```python
from build123d import *

# Parameters (mm, degrees)
EXTRUDE1_DEPTH                     = 2.5
SKETCH2_W                          = 1.54
SKETCH2_H                          = 0.508742985
CUT_EXTRUDE1_DEPTH                 = 12.5
SKETCH3_W                          = 0.65
SKETCH3_H                          = 0.65
EXTRUDE2_DEPTH                     = 3.54
CHAMFER1_SIZE                      = 0.35
CHAMFER1_SIZE2                     = 0.16320768
CHAMFER1_PART_2_SIZE               = 0.35
CHAMFER1_PART_2_SIZE2              = 0.16320768
CHAMFER1_PART_3_SIZE               = 0.35
CHAMFER1_PART_3_SIZE2              = 0.16320768
CHAMFER1_PART_4_SIZE               = 0.35
CHAMFER1_PART_4_SIZE2              = 0.16320768
SKETCH4_W                          = 0.65
SKETCH4_H                          = 0.65
EXTRUDE3_DEPTH                     = 6
CHAMFER2_SIZE                      = 0.35
CHAMFER2_SIZE2                     = 0.16320768
CHAMFER2_PART_2_SIZE               = 0.35
CHAMFER2_PART_2_SIZE2              = 0.16320768
CHAMFER2_PART_3_SIZE               = 0.35
CHAMFER2_PART_3_SIZE2              = 0.16320768
CHAMFER2_PART_4_SIZE               = 0.35
CHAMFER2_PART_4_SIZE2              = 0.16320768
LPATTERN3_COUNT                    = 2
LPATTERN3_PITCH                    = 2.54
LPATTERN3_COUNT_DIR2               = 2
LPATTERN3_PITCH_DIR2               = 2.54
LPATTERN4_COUNT                    = 2
LPATTERN4_PITCH                    = 2.54
LPATTERN4_COUNT_DIR2               = 2
LPATTERN4_PITCH_DIR2               = 2.54
CHAMFER1_OF_LPATTERN4_SIZE2        = 0.16320768
CHAMFER1_OF_LPATTERN4_SIZE         = 0.35
CHAMFER1_PART_2_OF_LPATTERN4_SIZE2 = 0.16320768
CHAMFER1_PART_2_OF_LPATTERN4_SIZE  = 0.35
CHAMFER1_PART_3_OF_LPATTERN4_SIZE2 = 0.16320768
CHAMFER1_PART_3_OF_LPATTERN4_SIZE  = 0.35
CHAMFER1_PART_4_OF_LPATTERN4_SIZE2 = 0.16320768
CHAMFER1_PART_4_OF_LPATTERN4_SIZE  = 0.35
CHAMFER2_OF_LPATTERN4_SIZE2        = 0.16320768
CHAMFER2_OF_LPATTERN4_SIZE         = 0.35
CHAMFER2_PART_2_OF_LPATTERN4_SIZE2 = 0.16320768
CHAMFER2_PART_2_OF_LPATTERN4_SIZE  = 0.35
CHAMFER2_PART_3_OF_LPATTERN4_SIZE2 = 0.16320768
CHAMFER2_PART_3_OF_LPATTERN4_SIZE  = 0.35
CHAMFER2_PART_4_OF_LPATTERN4_SIZE2 = 0.16320768
CHAMFER2_PART_4_OF_LPATTERN4_SIZE  = 0.35
ESBO_O1_R                          = 0.039608668
CORTE_EXTRUS_O1_DEPTH              = 0.1


with BuildPart() as part:
    # Sketch1 → Extrude1 (new body)
    with BuildSketch(Plane(origin=(0, 0, 0), x_dir=(1, 0, 0), z_dir=(0, 1, 0))):
        Polygon((-0.97, 1.27), (0.97, 1.27), (1.27, 0.97), (1.27, -0.97), (0.97, -1.27), (-0.97, -1.27), (-1.27, -0.97), (-1.27, 0.97), align=None)
    extrude1 = extrude(amount=EXTRUDE1_DEPTH)

    # Sketch2 → Cut-Extrude1 (cut)
    with BuildSketch(Plane.XY.offset(1.27)):
        with Locations((0, 2.314371493)):
            Rectangle(SKETCH2_W, SKETCH2_H)
    cut_extrude1 = extrude(amount=-CUT_EXTRUDE1_DEPTH, mode=Mode.SUBTRACT)

    # Sketch3 → Extrude2 (add)
    with BuildSketch(Plane(origin=(0, 2.06, 0), x_dir=(-1, 0, 0), z_dir=(0, 1, 0))):
        Rectangle(SKETCH3_W, SKETCH3_H)
    extrude2 = extrude(amount=EXTRUDE2_DEPTH)

    # Chamfer1
    chamfer1_edges = [part.edges().sort_by_distance(p)[0] for p in [
        (-0.325, 5.6, 0),
    ]]
    chamfer1_side = [part.faces().sort_by_distance(p)[0] for p in [
        (-0.325, 3.83, 0),
    ]]
    chamfer(chamfer1_edges, length=CHAMFER1_SIZE, length2=CHAMFER1_SIZE2, reference=chamfer1_side[0])

    # Chamfer1 part 2
    chamfer1_part_2_edges = [part.edges().sort_by_distance(p)[0] for p in [
        (0, 5.6, 0.325),
    ]]
    chamfer1_part_2_side = [part.faces().sort_by_distance(p)[0] for p in [
        (0, 3.83, 0.325),
    ]]
    chamfer(chamfer1_part_2_edges, length=CHAMFER1_PART_2_SIZE, length2=CHAMFER1_PART_2_SIZE2, reference=chamfer1_part_2_side[0])

    # Chamfer1 part 3
    chamfer1_part_3_edges = [part.edges().sort_by_distance(p)[0] for p in [
        (0.325, 5.6, 0),
    ]]
    chamfer1_part_3_side = [part.faces().sort_by_distance(p)[0] for p in [
        (0.325, 3.83, 0),
    ]]
    chamfer(chamfer1_part_3_edges, length=CHAMFER1_PART_3_SIZE, length2=CHAMFER1_PART_3_SIZE2, reference=chamfer1_part_3_side[0])

    # Chamfer1 part 4
    chamfer1_part_4_edges = [part.edges().sort_by_distance(p)[0] for p in [
        (0, 5.6, -0.325),
    ]]
    chamfer1_part_4_side = [part.faces().sort_by_distance(p)[0] for p in [
        (0, 3.83, -0.325),
    ]]
    chamfer(chamfer1_part_4_edges, length=CHAMFER1_PART_4_SIZE, length2=CHAMFER1_PART_4_SIZE2, reference=chamfer1_part_4_side[0])

    # Sketch4 → Extrude3 (add)
    with BuildSketch(Plane.XZ):
        Rectangle(SKETCH4_W, SKETCH4_H)
    extrude3 = extrude(amount=EXTRUDE3_DEPTH)

    # Chamfer2
    chamfer2_edges = [part.edges().sort_by_distance(p)[0] for p in [
        (-0.325, -6, 0),
    ]]
    chamfer2_side = [part.faces().sort_by_distance(p)[0] for p in [
        (-0.325, -3, 0),
    ]]
    chamfer(chamfer2_edges, length=CHAMFER2_SIZE, length2=CHAMFER2_SIZE2, reference=chamfer2_side[0])

    # Chamfer2 part 2
    chamfer2_part_2_edges = [part.edges().sort_by_distance(p)[0] for p in [
        (0, -6, -0.325),
    ]]
    chamfer2_part_2_side = [part.faces().sort_by_distance(p)[0] for p in [
        (0, -3, -0.325),
    ]]
    chamfer(chamfer2_part_2_edges, length=CHAMFER2_PART_2_SIZE, length2=CHAMFER2_PART_2_SIZE2, reference=chamfer2_part_2_side[0])

    # Chamfer2 part 3
    chamfer2_part_3_edges = [part.edges().sort_by_distance(p)[0] for p in [
        (0.325, -6, 0),
    ]]
    chamfer2_part_3_side = [part.faces().sort_by_distance(p)[0] for p in [
        (0.325, -3, 0),
    ]]
    chamfer(chamfer2_part_3_edges, length=CHAMFER2_PART_3_SIZE, length2=CHAMFER2_PART_3_SIZE2, reference=chamfer2_part_3_side[0])

    # Chamfer2 part 4
    chamfer2_part_4_edges = [part.edges().sort_by_distance(p)[0] for p in [
        (0, -6, 0.325),
    ]]
    chamfer2_part_4_side = [part.faces().sort_by_distance(p)[0] for p in [
        (0, -3, 0.325),
    ]]
    chamfer(chamfer2_part_4_edges, length=CHAMFER2_PART_4_SIZE, length2=CHAMFER2_PART_4_SIZE2, reference=chamfer2_part_4_side[0])

    # LPattern3: Extrude1, Cut-Extrude1 2 × 2
    with Locations(*[(-j * LPATTERN3_PITCH_DIR2, 0, -i * LPATTERN3_PITCH) for i in range(LPATTERN3_COUNT) for j in range(LPATTERN3_COUNT_DIR2) if (i, j) != (0, 0)]):
        add(extrude1)
        add(cut_extrude1, mode=Mode.SUBTRACT)

    # LPattern4: Extrude2, Extrude3 2 × 2
    with Locations(*[(-j * LPATTERN4_PITCH_DIR2, 0, -i * LPATTERN4_PITCH) for i in range(LPATTERN4_COUNT) for j in range(LPATTERN4_COUNT_DIR2) if (i, j) != (0, 0)]):
        add(extrude2)
        add(extrude3)

    # Chamfer1 of LPattern4
    chamfer1_of_lpattern4_edges = [part.edges().sort_by_distance(p)[0] for p in [
        (-2.865, 5.6, 0),
        (-0.325, 5.6, -2.54),
        (-2.865, 5.6, -2.54),
    ]]
    chamfer(chamfer1_of_lpattern4_edges, length=CHAMFER1_OF_LPATTERN4_SIZE, length2=CHAMFER1_OF_LPATTERN4_SIZE2)

    # Chamfer1 part 2 of LPattern4
    chamfer1_part_2_of_lpattern4_edges = [part.edges().sort_by_distance(p)[0] for p in [
        (-2.54, 5.6, 0.325),
        (0, 5.6, -2.215),
        (-2.54, 5.6, -2.215),
    ]]
    chamfer(chamfer1_part_2_of_lpattern4_edges, length=CHAMFER1_PART_2_OF_LPATTERN4_SIZE, length2=CHAMFER1_PART_2_OF_LPATTERN4_SIZE2)

    # Chamfer1 part 3 of LPattern4
    chamfer1_part_3_of_lpattern4_edges = [part.edges().sort_by_distance(p)[0] for p in [
        (-2.215, 5.6, 0),
        (0.325, 5.6, -2.54),
        (-2.215, 5.6, -2.54),
    ]]
    chamfer(chamfer1_part_3_of_lpattern4_edges, length=CHAMFER1_PART_3_OF_LPATTERN4_SIZE, length2=CHAMFER1_PART_3_OF_LPATTERN4_SIZE2)

    # Chamfer1 part 4 of LPattern4
    chamfer1_part_4_of_lpattern4_edges = [part.edges().sort_by_distance(p)[0] for p in [
        (-2.54, 5.6, -0.325),
        (0, 5.6, -2.865),
        (-2.54, 5.6, -2.865),
    ]]
    chamfer(chamfer1_part_4_of_lpattern4_edges, length=CHAMFER1_PART_4_OF_LPATTERN4_SIZE, length2=CHAMFER1_PART_4_OF_LPATTERN4_SIZE2)

    # Chamfer2 of LPattern4
    chamfer2_of_lpattern4_edges = [part.edges().sort_by_distance(p)[0] for p in [
        (-2.865, -6, 0),
        (-0.325, -6, -2.54),
        (-2.865, -6, -2.54),
    ]]
    chamfer(chamfer2_of_lpattern4_edges, length=CHAMFER2_OF_LPATTERN4_SIZE, length2=CHAMFER2_OF_LPATTERN4_SIZE2)

    # Chamfer2 part 2 of LPattern4
    chamfer2_part_2_of_lpattern4_edges = [part.edges().sort_by_distance(p)[0] for p in [
        (-2.54, -6, -0.325),
        (0, -6, -2.865),
        (-2.54, -6, -2.865),
    ]]
    chamfer(chamfer2_part_2_of_lpattern4_edges, length=CHAMFER2_PART_2_OF_LPATTERN4_SIZE, length2=CHAMFER2_PART_2_OF_LPATTERN4_SIZE2)

    # Chamfer2 part 3 of LPattern4
    chamfer2_part_3_of_lpattern4_edges = [part.edges().sort_by_distance(p)[0] for p in [
        (-2.215, -6, 0),
        (0.325, -6, -2.54),
        (-2.215, -6, -2.54),
    ]]
    chamfer(chamfer2_part_3_of_lpattern4_edges, length=CHAMFER2_PART_3_OF_LPATTERN4_SIZE, length2=CHAMFER2_PART_3_OF_LPATTERN4_SIZE2)

    # Chamfer2 part 4 of LPattern4
    chamfer2_part_4_of_lpattern4_edges = [part.edges().sort_by_distance(p)[0] for p in [
        (-2.54, -6, 0.325),
        (0, -6, -2.215),
        (-2.54, -6, -2.215),
    ]]
    chamfer(chamfer2_part_4_of_lpattern4_edges, length=CHAMFER2_PART_4_OF_LPATTERN4_SIZE, length2=CHAMFER2_PART_4_OF_LPATTERN4_SIZE2)

    # Esboço1 → Corte-extrusão1 (cut)
    with BuildSketch(Plane(origin=(0, 5.6, 0), x_dir=(1, 0, 0), z_dir=(0, 1, 0))):
        Circle(ESBO_O1_R)
    extrude(amount=-CORTE_EXTRUS_O1_DEPTH, mode=Mode.SUBTRACT)


solid = part.part
```
Design review of the part built by this model. Coordinates are the model's own, in mm. A direction names the side the tool comes from. Coordinates: 2 decimals unless noted, no trailing zeros. Order: outer loops, then holes, each group sorted by start corner. A loop starts at its lowest first (then second) coordinate and runs counter-clockwise, first axis right, second up.
1) Take a section at A-A, the plane y = -1.75. Give the boundary of the cut face in (x, z) (3 decimals).
2) Mouldability with a two-part tool opening along X and no side actions: class faces 3 (the flat face through (-3.81, 1, -3)), 4 (the flat face through (0, 2.06, -1)), 5 (the flat face through (0, 1, -3.81)) as +X half, -X half, draft (parallel to the pull), parting line (faces both ways), or undercut.
3) Clearance check with flat-ended pins moving along their axes: pin 1 (1 mm diameter, centred on x = -2, z = -1, fed in from +Y); pin 2 (0.7 mm diameter, centred on y = 4, z = -2.5, fed in from -X) (3 decimals); pin 3 (1.2 mm diameter, centred on x = -3, z = -2.5, fed in from +Y); pin 4 (0.7 mm diameter, centred on x = -2.5, y = -3, fed in from +Z) (3 decimals). State where each tip first meets the part, or that it passes through.
4) Take a section at B-B, the plane y = 0.25. Give the boundary of the cut face in (x, z), and give its area (3 significant figures).
5) Take a section at D-D, the plane z = -3.4. Give the boundary of the cut face in (x, y).
6) Wall thickness on line 1 along X through (y, z) = (3.5, 0) (3 decimals); line 2 along Y through (x, z) = (-1, -1.2): over which ranges is each line inside the solid? List them lowest first.
7) Take a section at C-C, the plane z = -1.15. Give the boundary of the cut face in (x, y), and give its area (3 significant figures).
8) For faces 1 (the flat face through (-3.81, 1, 0)), 2 (the flat face through (-1, 2.5, -1)), list the 3-axis set-ups (+Z, -Z, +X, -X, +Y, -Y) from which the entire face can be reached by the end or side of a thin tool; tool diameter is ignored.
Returned:
1. outline: (-2.865, -2.865) - (-2.215, -2.865) - (-2.215, -2.215) - (-2.865, -2.215) - close; (-2.865, -0.325) - (-2.215, -0.325) - (-2.215, 0.325) - (-2.865, 0.325) - close; (-0.325, -2.865) - (0.325, -2.865) - (0.325, -2.215) - (-0.325, -2.215) - close; (-0.325, -0.325) - (0.325, -0.325) - (0.325, 0.325) - (-0.325, 0.325) - close
2. face 3: -X half
2. face 4: undercut
2. face 5: draft
3. pin 1: stops at y = 2.5
3. pin 2: stops at x = -2.865
3. pin 3: stops at y = 5.6
3. pin 4: stops at z = 0.325
4. outline: (-3.81, -3.51) - (-3.51, -3.81) - (-1.57, -3.81) - (-1.27, -3.51) - (-0.97, -3.81) - (0.97, -3.81) - (1.27, -3.51) - (1.27, -1.57) - (0.97, -1.27) - (1.27, -0.97) - (1.27, 0.97) - (0.97, 1.27) - (-0.97, 1.27) - (-1.27, 0.97) - (-1.57, 1.27) - (-3.51, 1.27) - (-3.81, 0.97) - (-3.81, -0.97) - (-3.51, -1.27) - (-3.81, -1.57) - close; hole (-1.57, -1.27) - (-1.27, -1.57) - (-0.97, -1.27) - (-1.27, -0.97) - close
4. area: 25.1 mm2
5. outline: (-3.81, 0) - (1.27, 0) - (1.27, 2.5) - (0.77, 2.5) - (0.77, 2.06) - (-0.77, 2.06) - (-0.77, 2.5) - (-1.77, 2.5) - (-1.77, 2.06) - (-3.31, 2.06) - (-3.31, 2.5) - (-3.81, 2.5) - close
6. line 1: x = -2.865 to -2.215, -0.325 to 0.325
6. line 2: y = 0 to 2.5
7. outline: (-3.63, 0) - (-1.45, 0) - (-1.45, 2.5) - (-1.77, 2.5) - (-1.77, 2.06) - (-3.31, 2.06) - (-3.31, 2.5) - (-3.63, 2.5) - close; (-1.09, 0) - (1.09, 0) - (1.09, 2.5) - (0.77, 2.5) - (0.77, 2.06) - (-0.77, 2.06) - (-0.77, 2.5) - (-1.09, 2.5) - close
7. area: 9.54 mm2
8. face 1: +Z, -Z, -X, +Y, -Y
8. face 2: +Z, -Z, +Y
